from build123d import *

# Parameters (mm, degrees)
F0_R     = 25.4
F1_DEPTH = 50.8


with BuildPart() as f1:
    # F0 (on Front) → F1 (new body)
    with BuildSketch(Plane.XZ):
        with BuildLine():
            ThreePointArc((-148.411867, 727.363636), (-108.530539, 381), (-148.411867, 34.636364))
            ThreePointArc((-148.411867, 34.636364), (0, -152.4), (148.411867, 34.636364))
            ThreePointArc((148.411867, 34.636364), (108.530539, 381), (148.411867, 727.363636))
            ThreePointArc((148.411867, 727.363636), (0, 914.4), (-148.411867, 727.363636))
        make_face()
        Circle(F0_R, mode=Mode.SUBTRACT)
        with Locations((0, 762)):
            Circle(F0_R, mode=Mode.SUBTRACT)
    extrude(amount=F1_DEPTH)


solid = f1.part
CAD build for the part. Positions are in the model's coordinates, mm. Round coordinates to 2 decimals unless told otherwise and drop trailing zeros. Write each loop counter-clockwise with the first axis right and the second up, starting at its lowest first coordinate (ties: lowest second). Pieces come first, ordered by that corner, then holes.
(1) Slice it at B-B, the plane z = 762. Write the cut outline in (x, y), and give its area (3 significant figures).
(2) Mould opens along Z. For faces 1 (the face through (-2, 0, 388)), 2 (the face through (-3.307, -25.044, 787.184)) say: pulls with the +Z half, pulls with the -Z half, needs draft (parallel to the pull), parting line crosses it, or undercut.
(3) Slice it at D-D, the plane z = 127.5. Write the cut outline in (x, y).
(4) Slice it at C-C, the plane y = -31. Write the cut outline in (x, z).
(5) Probe line 1 along Z through (x, y) = (0, -35); line 2 along X through (y, z) = (-45.5, 760); line 3 along Z through (x, y) = (17, -5.5). List the from-to ranges inside material, lowest first.
(6) Slice it at A-A, the plane x = 0. Write the cut outline in (y, z).
(7) Drop flat-ended pins along their axis: P1, Ø6, axis at x = -97, y = -20, coming from the +Z side; P2, Ø2, axis at y = -42.5, z = 472.5, coming from the -X side; P3, Ø4, axis at x = 91.5, y = -41.5, coming from the -Z side. Give the stop position or say it passes through.
From the geometry:
1. outline: (-152.4, -50.8) - (-25.4, -50.8) - (-25.4, 0) - (-152.4, 0) - close; (25.4, -50.8) - (152.4, -50.8) - (152.4, 0) - (25.4, 0) - close
1. area: 12,900 mm2
2. face 1: needs draft
2. face 2: undercut
3. outline: (-129.76, -50.8) - (129.76, -50.8) - (129.76, 0) - (-129.76, 0) - close
4. outline: (-148.41, 34.64) arc R152.4 ccw (long way) to (148.41, 34.64) arc R1524 cw to (148.41, 727.36) arc R152.4 ccw (long way) to (-148.41, 727.36) arc R1524 cw to start; hole circle Ø50.8 at (0, 0); hole circle Ø50.8 at (0, 762)
5. line 1: z = -152.4 to -25.4, 25.4 to 736.6, 787.4 to 914.4
5. line 2: x = -152.39 to -25.32, 25.32 to 152.39
5. line 3: z = -151.45 to -18.87, 18.87 to 743.13, 780.87 to 913.45
6. outline: (-50.8, -152.4) - (0, -152.4) - (0, -25.4) - (-50.8, -25.4) - close; (-50.8, 25.4) - (0, 25.4) - (0, 736.6) - (-50.8, 736.6) - close; (-50.8, 787.4) - (0, 787.4) - (0, 914.4) - (-50.8, 914.4) - close
7. P1: stops at z = 881.96
7. P2: stops at x = -111.34
7. P3: stops at z = -123.35
